from build123d import *

# Parameters (mm, degrees)
SKETCH2_R               = 7
BOSS_EXTRUDE1_DEPTH     = 55
CUT_EXTRUDE1_DEPTH      = 1
CUT_EXTRUDE1_DEPTH_BACK = 20
SKETCH5_W               = 25
SKETCH5_H               = 18
CUT_EXTRUDE2_DEPTH      = 91


with BuildPart() as part:
    # Sketch2 → Boss-Extrude1 (new body)
    with BuildSketch(Plane.XY):
        Polygon((0, 0), (0, 35), (20, 60), (35, 35), (35, 12), (60, 12), (60, 25), (90, 25), (90, 0), align=None)
        with Locations((20, 20)):
            Circle(SKETCH2_R, mode=Mode.SUBTRACT)
    extrude(amount=BOSS_EXTRUDE1_DEPTH)

    # Sketch3 → Cut-Extrude1 (cut, two sides)
    with BuildSketch(Plane(origin=(90, 0, 0), x_dir=(0, 0, -1), z_dir=(1, 0, 0))) as cut_extrude1_sk:
        Polygon((-203.084488957, -69.042244479), (-55, 5), (-15, 25), (133.084488957, 99.042244479), (-15, 395.211222394), (-351.168977915, 227.126733436), align=None)
    extrude(amount=CUT_EXTRUDE1_DEPTH, mode=Mode.SUBTRACT)
    extrude(cut_extrude1_sk.sketch, amount=-CUT_EXTRUDE1_DEPTH_BACK, mode=Mode.SUBTRACT)

    # Sketch5 → Cut-Extrude2 (cut, through all)
    with BuildSketch(Plane.ZY):
        with Locations((27.5, 51)):
            Rectangle(SKETCH5_W, SKETCH5_H)
    extrude(amount=-CUT_EXTRUDE2_DEPTH, mode=Mode.SUBTRACT)


solid = part.part
The model under review builds one solid part; all positions refer to its coordinate system, in mm. A direction names the side the tool comes from. Coordinates: 2 decimals unless noted, no trailing zeros. Write each loop counter-clockwise with the first axis right and the second up, starting at its lowest first coordinate (ties: lowest second). Pieces come first, ordered by that corner, then holes. Notation, with made-up numbers: (14, 87.25) - (24, 87.25) arc R23 ccw to (24, 115.25) - close; hole circle Ø8 at (6.25, 9). An arc over 180 degrees is marked (long way). Answer as a JSON object with one key per item and string values. Group by question number.
1. Add section C-C (x = 9). Give the boundary of the cut face in (y, z).
2. Clearance check with flat-ended pins moving along their axes: pin 1 Ø5.5 at (x, y) = (14.5, 47) entering from -Z; pin 2 Ø2 at (x, z) = (72, 9.5) entering from +Y; pin 3 Ø15 at (x, z) = (82, 28) entering from +Y; pin 4 Ø12.5 at (x, y) = (20, 20) entering from +Z. State where each tip first meets the part, or that it passes through.
3. Mouldability with a two-part tool opening along Z and no side actions: class faces 4 (the face through (18, 47, 15)), 5 (the face through (5.416, 41.769, 27.115)), 6 (the face through (80, 15, 35)) as pulls with the +Z half, pulls with the -Z half, needs draft (parallel to the pull), parting line crosses it, or undercut.
4. To check wall thickness, follow probe 1 along X at (y, z) = (12.5, 15); probe 2 along Y at (x, z) = (20, 17); probe 3 along Y at (x, z) = (41.5, 21.5). State the ranges of each line that lie inside material, in increasing order.
5. Add section D-D (z = 33). Give the boundary of the cut face in (x, y), plus the area to 3 significant figures.
6. Add section B-B (z = 49.5). Give the boundary of the cut face in (x, y), plus the area to 3 significant figures.
7. Add section A-A (y = 20). Give the boundary of the cut face in (x, z), plus the area to 4 significant figures.
8. Machinability: for faces 1 (the face through (60, 18, 27)), 2 (the face through (70, 17, 40)), 3 (the face through (68, 25, 21)), which of the approach directions +Z, -Z, +X, -X, +Y, -Y give a long, thin tool a straight path to every point of the face, cutting with its end or side? Answer none if there is none.
Findings:
{
 "1": {"outline": "(0, 0) - (46.25, 0) - (46.25, 15) - (42, 15) - (42, 40) - (46.25, 40) - (46.25, 55) - (0, 55) - close"},
 "2": {"pin 1": "z = 0", "pin 2": "y = 25", "pin 3": "y = 22.25", "pin 4": "through"},
 "3": {"face 4": "undercut", "face 5": "needs draft", "face 6": "pulls with the +Z half"},
 "4": {"probe 1": "0 to 35, 60 to 90", "probe 2": "0 to 13, 27 to 42", "probe 3": "0 to 12"},
 "5": {"outline": "(0, 0) - (90, 0) - (90, 16) - (70, 16) - (70, 25) - (60, 25) - (60, 12) - (35, 12) - (35, 35) - (30.8, 42) - (5.6, 42) - (0, 35) - close; hole circle Ø14 at (20, 20)", "area": "2,150 mm²"},
 "6": {"outline": "(0, 0) - (90, 0) - (90, 7.75) - (70, 7.75) - (70, 25) - (60, 25) - (60, 12) - (35, 12) - (35, 35) - (20, 60) - (0, 35) - close; hole circle Ø14 at (20, 20)", "area": "2,210 mm²"},
 "7": {"outline": "(0, 0) - (13, 0) - (13, 55) - (0, 55) - close; (27, 0) - (35, 0) - (35, 55) - (27, 55) - close; (60, 0) - (90, 0) - (90, 25) - (70, 25) - (70, 55) - (60, 55) - close", "area": "2,205 mm²"},
 "8": {"face 1": "+Z, -Z, +Y", "face 2": "+Z, +X, +Y", "face 3": "+Z, -Z, +X, +Y"}
}
